```python
from build123d import *

# Parameters (mm, degrees)
SKETCH2_R           = 22.5
BOSS_EXTRUDE1_DEPTH = 3
SKETCH3_R           = 10
SKETCH3_R_2         = 7
BOSS_EXTRUDE2_DEPTH = 15
SKETCH1_R           = 1.5
CUT_EXTRUDE1_DEPTH  = 9


with BuildPart() as part:
    # Sketch2 → Boss-Extrude1 (new body)
    with BuildSketch(Plane.XY):
        with Locations((0, 10)):
            Circle(SKETCH2_R)
    extrude(amount=BOSS_EXTRUDE1_DEPTH)

    # Sketch3 → Boss-Extrude2 (add)
    with BuildSketch(Plane(origin=(0, 0, 0), x_dir=(-1, 0, 0), z_dir=(0, 0, -1))):
        with Locations(Location((0, 10, 0), (0, 0, 180))):
            Circle(SKETCH3_R)
        with Locations((0, 10)):
            Circle(SKETCH3_R_2, mode=Mode.SUBTRACT)
    extrude(amount=BOSS_EXTRUDE2_DEPTH)

    # Sketch1 → Cut-Extrude1 (cut)
    with BuildSketch(Plane.XY):
        with Locations((0, 25)):
            Circle(SKETCH1_R)
        with Locations((15, 10)):
            Circle(SKETCH1_R)
        with Locations((0, -5)):
            Circle(SKETCH1_R)
        with Locations((-15, 10)):
            Circle(SKETCH1_R)
    extrude(amount=CUT_EXTRUDE1_DEPTH, mode=Mode.SUBTRACT)


solid = part.part
```
The listing builds one solid part. Answer for the finished solid, in the listing's coordinates (mm). A direction names the side the tool comes from. Coordinates: 2 decimals unless noted, no trailing zeros. Loops run counter-clockwise (first coordinate to the right, second up) from the corner with the lowest first, then second, coordinate; pieces in that order, holes last. Notation, with made-up numbers: (-15, 16.25) -> (33, 16.25) arc R24 cw to (33, 54.25) -> close; hole circle Ø7 at (83, -28). An arc over 180 degrees is marked (long way). Return JSON: item names as keys, results as strings. Group by question number.
(1) Find the intervals of material crossed by probe 1 along Y at (x, z) = (0, 1.15); probe 2 along Z at (x, y) = (-18, 0); probe 3 along X at (y, z) = (-5, 1.8), in increasing order. Write a range as from..to.
(2) A cutting plane is placed at D-D on x = -15. Write down the section's boundary in (y, z).
(3) A cutting plane is placed at A-A on x = 0. Write down the section's boundary in (y, z).
(4) Given pin 1 Ø1 at (y, z) = (12.5, -4) entering from -X; pin 2 Ø4 at (y, z) = (4, -9.5) entering from +X; pin 3 Ø2 at (x, y) = (15.5, 16) entering from -Z, each flat-ended and moving along its own axis, determine where each tip first touches the part or whether it passes through.
(5) Determine the mould class of faces 1 (the cylindrical face through (-4.878, -11.965, 1.479)), 2 (the cylindrical face through (13.5, 10.07, 1.48)), 3 (the flat face through (0, 10, 3)) for opening direction Y: released by +Y, released by -Y, zero draft, split by the parting line, or undercut.
(6) A cutting plane is placed at C-C on z = 0.75. Write down the section's boundary in (x, y), and give its area (3 significant figures).
(7) Which of the six approach directions +Z, -Z, +X, -X, +Y, -Y give full straight-line access (tool end or side, diameter ignored) to faces 4 (the flat face through (-7, 12, -15)), 5 (the cylindrical face through (-8, 16, -7))?
(8) A cutting plane is placed at B-B on y = 10. Write down the section's boundary in (x, z).
The answers:
{
 "1": {"probe 1": "y = -12.5..-6.5, -3.5..23.5, 26.5..32.5", "probe 2": "z = 0..3", "probe 3": "x = -16.77..-1.5, 1.5..16.77"},
 "2": {"outline": "(-6.77, 0) -> (8.5, 0) -> (8.5, 3) -> (-6.77, 3) -> close; (11.5, 0) -> (26.77, 0) -> (26.77, 3) -> (11.5, 3) -> close"},
 "3": {"outline": "(-12.5, 0) -> (-6.5, 0) -> (-6.5, 3) -> (-12.5, 3) -> close; (-3.5, 0) -> (0, 0) -> (0, -15) -> (3, -15) -> (3, 0) -> (17, 0) -> (17, -15) -> (20, -15) -> (20, 0) -> (23.5, 0) -> (23.5, 3) -> (-3.5, 3) -> close; (26.5, 0) -> (32.5, 0) -> (32.5, 3) -> (26.5, 3) -> close"},
 "4": {"pin 1": "stops at x = -9.8", "pin 2": "stops at x = 9.17", "pin 3": "stops at z = 0"},
 "5": {"face 1": "split by the parting line", "face 2": "undercut", "face 3": "zero draft"},
 "6": {"outline": "circle Ø45 at (0, 10); hole circle Ø3 at (-15, 10); hole circle Ø3 at (0, -5); hole circle Ø3 at (0, 25); hole circle Ø3 at (15, 10)", "area": "1,560 mm^2"},
 "7": {"face 4": "-Z, +X, -X, +Y, -Y", "face 5": "-Z"},
 "8": {"outline": "(-22.5, 0) -> (-16.5, 0) -> (-16.5, 3) -> (-22.5, 3) -> close; (-13.5, 0) -> (-10, 0) -> (-10, -15) -> (-7, -15) -> (-7, 0) -> (7, 0) -> (7, -15) -> (10, -15) -> (10, 0) -> (13.5, 0) -> (13.5, 3) -> (-13.5, 3) -> close; (16.5, 0) -> (22.5, 0) -> (22.5, 3) -> (16.5, 3) -> close"}
}
